Geometry: final body of the model. Coordinates: model frame, mm. Face numbers are marked on the shaded views. Coordinates: 2 decimals unless noted, no trailing zeros. Write each loop counter-clockwise with the first axis right and the second up, starting at its lowest first coordinate (ties: lowest second). Pieces come first, ordered by that corner, then holes. Notation, with made-up numbers: (53.5, 87.25) -> (100.5, 87.25) arc R5 ccw to (100.5, 94.25) -> close; hole circle Ø10 at (6, 1). An arc over 180 degrees is marked (long way). One line per item, written item: value.
Autodesk Fusion 360 part; units mm, degrees
sketch "Sketch1" plane through (0, 0, 0) normal (0, 0, 1) x (1, 0, 0)
  line L0 (0, 0) -> (0, 50) construction
  line L1 (7, 50) -> (14, 50)
  line L2 (14, 50) -> (14, 10)
  line L3 (14, 10) -> (19, 0)
  line L4 (19, 0) -> (7, 0)
  line L5 (7, 0) -> (7, 50)
  line L6 (0, 47) -> (7, 47)
  line L7 (7, 47) -> (7, 50)
  line L8 (7, 50) -> (14, 50)
  line L9 (14, 50) -> (14, 44)
  line L10 (14, 44) -> (20, 44)
  line L11 (20, 44) -> (20, 47)
  arc A0 (20, 47) -> (10, 57) centre (10, 47) ccw
  line L12 (10, 57) -> (0, 57)
  line L13 (0, 57) -> (0, 47)
  dimension "d1" = 50
  dimension "d2" = 7
  dimension "d3" = 14
  dimension "d4" = 12
  dimension "d5" = 10
  dimension "d7" = 3
  dimension "d8" = 6
  dimension "d9" = 3
  dimension "d10" = 10
  dimension "d11" = 10
  dimension "d12" = 20
revolve "Revolve1" add sketch "Sketch1" angle 360 about axis through (0, 0, 0) along (0, 1, 0) contours L1 L2 L3 L4 L5 L7 L8 L9
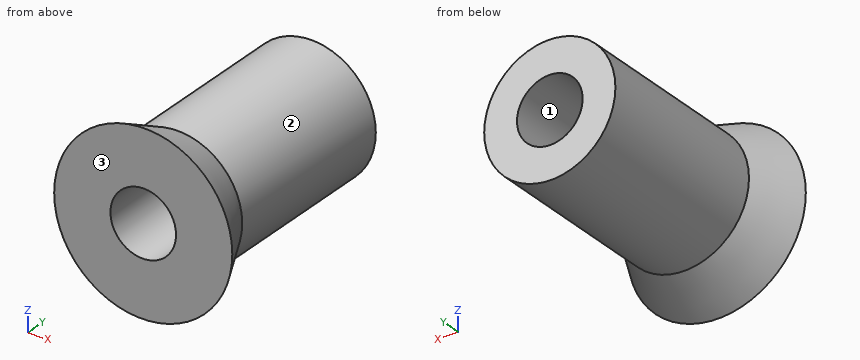
(1) First-contact query: pin 1 (5 mm diameter, centred on y = 19.5, z = -12, fed in from -X); pin 2 (8.5 mm diameter, centred on x = 0, z = 0, fed in from -Y); pin 3 (12 mm diameter, centred on y = 41.5, z = 8.5, fed in from +X) (3 decimals); pin 4 (4 mm diameter, centred on x = 12, y = 24, fed in from -Z). Flat tips, straight axial feed; report the tip coordinate or a pass-through.
Responses:
pin 1: stops at x = -10.28
pin 2: passes through
pin 3: stops at x = 13.775
pin 4: stops at z = -9.8
(2) Line query: line 1 (X direction, y = 21.5, z = 0); line 2 (X direction, y = 40.5, z = 2). Output: solid intervals per line, ascending. Write a range as [from, to].
Responses:
line 1: x = [-14, -7], [7, 14]
line 2: x = [-13.86, -6.71], [6.71, 13.86]
(3) Section A-A (x = 0). Return the cut outline in (y, z), then the cut area to 3 significant figures.
Responses:
outline: (0, -19) -> (10, -14) -> (50, -14) -> (50, -7) -> (0, -7) -> close; (0, 7) -> (50, 7) -> (50, 14) -> (10, 14) -> (0, 19) -> close
area: 750 mm2
(4) Pull-direction query (Z, two-part tool) for the marked faces 1, 2 and 3; classes: released by +Z, released by -Z, zero draft, split by the parting line, or undercut.
Responses:
face 1: undercut
face 2: split by the parting line
face 3: zero draft
(5) Section C-C (y = 29). Return the cut outline in (x, z).
Responses:
outline: circle Ø28 at (0, 0); hole circle Ø14 at (0, 0)
(6) Section B-B (z = 0). Return the cut outline in (x, y).
Responses:
outline: (-19, 0) -> (-7, 0) -> (-7, 50) -> (-14, 50) -> (-14, 10) -> close; (7, 0) -> (19, 0) -> (14, 10) -> (14, 50) -> (7, 50) -> close
